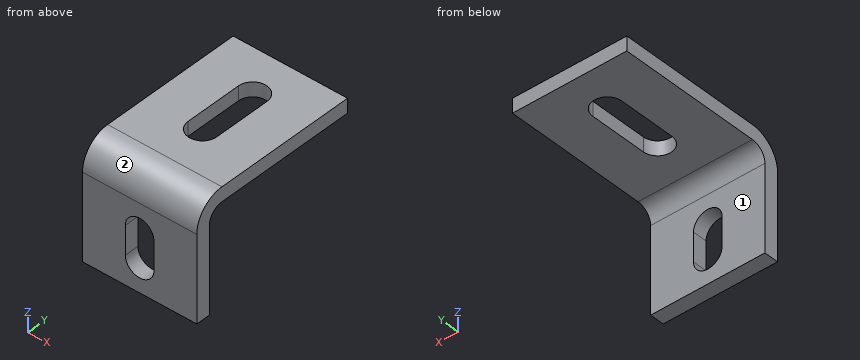
```python
from build123d import *

# Parameters (mm, degrees)
EXTRUDE_THIN1_DEPTH = 12.7
CUT_EXTRUDE1_DEPTH  = 44.301226888
CUT_EXTRUDE2_DEPTH  = 44.301226888


with BuildPart() as part:
    # Sketch4 → Extrude-Thin1 (new, symmetric)
    with BuildSketch(Plane(origin=(0, 0, 0), x_dir=(0, 0, -1), z_dir=(1, 0, 0))):
        with BuildLine():
            Line((-3.175, 34.925), (-3.175, 3.175))
            ThreePointArc((-3.175, 3.175), (-1.315128061, -1.315128061), (3.175, -3.175))
            Line((3.175, -3.175), (22.225, -3.175))
            Line((22.225, -3.175), (22.225, 0))
            Line((22.225, 0), (3.175, 0))
            ThreePointArc((3.175, 0), (0.92993597, 0.92993597), (0, 3.175))
            Line((0, 3.175), (0, 34.925))
            Line((0, 34.925), (-3.175, 34.925))
        make_face()
    extrude(amount=EXTRUDE_THIN1_DEPTH, both=True)

    # Sketch5 → Cut-Extrude1 (cut, through all)
    with BuildSketch(Plane.XY):
        with BuildLine():
            Line((3.175, 25.4), (3.175, 12.7))
            ThreePointArc((3.175, 12.7), (0, 9.525), (-3.175, 12.7))
            Line((-3.175, 12.7), (-3.175, 25.4))
            ThreePointArc((-3.175, 25.4), (0, 28.575), (3.175, 25.4))
        make_face()
    extrude(amount=CUT_EXTRUDE1_DEPTH, mode=Mode.SUBTRACT)

    # Sketch6 → Cut-Extrude2 (cut, through all)
    with BuildSketch(Plane(origin=(0, 0, 0), x_dir=(1, 0, 0), z_dir=(0, 1, 0))):
        with BuildLine():
            Line((-3.175, 15.875), (-3.175, 9.525))
            ThreePointArc((-3.175, 9.525), (0, 6.35), (3.175, 9.525))
            Line((3.175, 9.525), (3.175, 15.875))
            ThreePointArc((3.175, 15.875), (0, 19.05), (-3.175, 15.875))
        make_face()
    extrude(amount=-CUT_EXTRUDE2_DEPTH, mode=Mode.SUBTRACT)


solid = part.part
```
Build history of the part. All positions in model axes, mm. Face numbers are marked on the shaded views. A direction names the side the tool comes from. Give positions to 0.01 mm unless a question says otherwise; leave off trailing zeros. Order: outer loops, then holes, each group sorted by start corner. A loop starts at its lowest first (then second) coordinate and runs counter-clockwise, first axis right, second up. Notation, with made-up numbers: M 79,-17 L 121,-17 A20 cw 121,21 Z; hole C 26.25,-12 d2. An arc over 180 degrees is marked long. Return JSON: item names as keys, results as strings.
Q1. Flat gauge pins, fed straight in: pin 1 (5.5 mm diameter, centred on x = 0, z = -17, fed in from +Y); pin 2 (1.5 mm diameter, centred on x = 6, y = 23, fed in from -Z); pin 3 (10 mm diameter, centred on x = -7, z = -2, fed in from +Y) (3 decimals). Where does each tip first touch, or does it go through?
Answer list:
{"pin 1": "stops at y = 0", "pin 2": "stops at z = 0", "pin 3": "stops at y = 34.925"}
Q2. Wall check: probe 1 along Y at (x, z) = (-3.25, -20.25) (3 decimals); probe 2 along Z at (x, y) = (-10.5, 29.5) (3 decimals); probe 3 along Z at (x, y) = (0.75, -1) (3 decimals). Give the ranges that are in metal, low to high. Write a range as from..to.
Answer list:
{"probe 1": "y = -3.175..0", "probe 2": "z = 0..3.175", "probe 3": "z = -22.225..-18.96, -6.44..1.61"}
Q3. 3-axis set-ups, long thin cutter, end or side, ignore diameter. For the marked faces 1 and 2: which of +Z, -Z, +X, -X, +Y, -Y reach the whole face in a straight line?
Answer list:
{"face 1": "-Z, +X, -X, +Y", "face 2": "+Z, +X, -X, -Y"}
Q4. Band-saw the part on D-D (x = -7). Give the cut face in (y, z) (3 decimals).
Answer list:
{"outline": "M -3.175,-22.225 L 0,-22.225 L 0,-3.175 A3.175 cw 3.175,0 L 34.925,0 L 34.925,3.175 L 3.175,3.175 A6.35 ccw -3.175,-3.175 Z"}
Q5. Band-saw the part on A-A (y = 16). Give the cut face in (x, z) (3 decimals).
Answer list:
{"outline": "M -12.7,0 L -3.175,0 L -3.175,3.175 L -12.7,3.175 Z; M 3.175,0 L 12.7,0 L 12.7,3.175 L 3.175,3.175 Z"}
Q6. Band-saw the part on B-B (x = 0). Give the cut face in (y, z) (3 decimals).
Answer list:
{"outline": "M -3.175,-22.225 L 0,-22.225 L 0,-19.05 L -3.175,-19.05 Z; M -3.175,-6.35 L 0,-6.35 L 0,-3.175 A3.175 cw 3.175,0 L 9.525,0 L 9.525,3.175 L 3.175,3.175 A6.35 ccw -3.175,-3.175 Z; M 28.575,0 L 34.925,0 L 34.925,3.175 L 28.575,3.175 Z"}
Q7. Band-saw the part on C-C (z = -8.25). Give the cut face in (x, y) (3 decimals).
Answer list:
{"outline": "M -12.7,-3.175 L -2.908,-3.175 L -2.908,0 L -12.7,0 Z; M 2.908,-3.175 L 12.7,-3.175 L 12.7,0 L 2.908,0 Z"}
